Geometry: final body of the model. Coordinates: model frame, mm. A direction names the side the tool comes from. Coordinates: 2 decimals unless noted, no trailing zeros. Write each loop counter-clockwise with the first axis right and the second up, starting at its lowest first coordinate (ties: lowest second). Pieces come first, ordered by that corner, then holes.
from build123d import *

# Parameters (mm, degrees)
ESQUISSE1_R                  = 4
BOSS_EXTRU_1_DEPTH           = 4
ESQUISSE2_R                  = 11
BOSS_EXTRU_2_DEPTH           = 5
ESQUISSE3_R                  = 2.1
ENL_V_MAT_EXTRU_1_DEPTH      = 18.972200756
TROU_TARAUD_M41_D            = 3.3
ESQUISSE6_R                  = 1.25
ENL_V_MAT_EXTRU_2_DEPTH      = 18.972200756
R_P_TITION_CIRCULAIRE1_COUNT = 2
R_P_TITION_CIRCULAIRE1_ANGLE = 90
CHANFREIN1_SIZE              = 0.5


with BuildPart() as part:
    # Esquisse1 → Boss.-Extru.1 (new body)
    with BuildSketch(Plane.XY):
        Circle(ESQUISSE1_R)
    extrude(amount=BOSS_EXTRU_1_DEPTH)

    # Esquisse2 → Boss.-Extru.2 (add)
    with BuildSketch(Plane.XY.offset(4)):
        Circle(ESQUISSE2_R)
    extrude(amount=BOSS_EXTRU_2_DEPTH)

    # Esquisse3 → Enlèv. mat.-Extru.1 (cut, through all)
    with BuildSketch(Plane.XY.offset(9)):
        with Locations((-5.656854249, 5.656854249)):
            Circle(ESQUISSE3_R)
        with Locations((5.656854249, -5.656854249)):
            Circle(ESQUISSE3_R)
        Circle(ESQUISSE3_R)
    extrude(amount=-ENL_V_MAT_EXTRU_1_DEPTH, mode=Mode.SUBTRACT)

    # Trou taraudé M41 (through all)
    with Locations(Plane.XY.offset(9)):
        with Locations((5.656854249, 5.656854249), (-5.656854249, -5.656854249)):
            Hole(TROU_TARAUD_M41_D / 2)

    # Esquisse6 → Enlèv. mat.-Extru.2 (cut, through all)
    with BuildSketch(Plane(origin=(0, 0, 0), x_dir=(1, 0, 0), z_dir=(0, 1, 0))):
        with Locations(Location((0, -6.5, 0), (0, 0, 270))):
            Circle(ESQUISSE6_R)
    enl_v_mat_extru_2 = extrude(amount=-ENL_V_MAT_EXTRU_2_DEPTH, mode=Mode.SUBTRACT)

    # Répétition circulaire1: Enlèv. mat.-Extru.2 ×2 about axis
    r_p_tition_circulaire1_axis = Axis((0, 0, 9), (0, 0, 1))
    for i in range(1, R_P_TITION_CIRCULAIRE1_COUNT):
        add(enl_v_mat_extru_2.rotate(r_p_tition_circulaire1_axis, i * R_P_TITION_CIRCULAIRE1_ANGLE / (R_P_TITION_CIRCULAIRE1_COUNT - 1)), mode=Mode.SUBTRACT)

    # Chanfrein1
    chanfrein1_edges = [part.edges().sort_by_distance(p)[0] for p in [
        (-4, 0, 0),
        (-11, 0, 4),
        (-11, 0, 9),
    ]]
    chamfer(chanfrein1_edges, length=CHANFREIN1_SIZE)


solid = part.part
Item 1: Material intervals for probe 1 along Y at (x, z) = (0, 3.25); probe 2 along X at (y, z) = (-5.75, 5); probe 3 along Y at (x, z) = (-6, 5.5), sorted ascending.
Derived:
probe 1: y = -4 to -2.1, 2.1 to 4
probe 2: x = -9.38 to -7.3, -4.01 to 3.56, 7.75 to 9.38
probe 3: y = -9.22 to -7.27, -4.04 to 3.59, 7.73 to 9.22
Item 2: Pull-direction query (X, two-part tool) for faces 1 (the cylindrical face through (-2.38, -10.74, 6.47)), 2 (the cylindrical face through (5.202, -7.707, 6.535)), 3 (the flat face through (2, -2, 0)); classes: released by +X, released by -X, zero draft, split by the parting line, or undercut.
Derived:
face 1: split by the parting line
face 2: undercut
face 3: zero draft
Item 3: Section D-D, the plane z = 2.5. Output: boundary loops of the cut face in (x, y), plus the area to 3 significant figures.
Derived:
outline: circle Ø8 at (0, 0); hole circle Ø4.2 at (0, 0)
area: 36.4 mm2
Item 4: Pin query (flat end, axial travel): pin 1 (2 mm diameter, centred on x = 0, z = 6.5, fed in from -Y); pin 2 (5 mm diameter, centred on y = -6, z = 3.5, fed in from -X); pin 3 (1 mm diameter, centred on x = -6.5, y = 0.5, fed in from -Z). Return the tip coordinate at first contact, or that it passes through.
Derived:
pin 1: stops at y = 1.85
pin 2: stops at x = -10.36
pin 3: stops at z = 4
Item 5: Set-up query: faces 4 (the flat face through (-0.1, 2.5, 9)), 5 (the cylindrical face through (6.28, 0.05, 5.25)), 6 (the cylindrical face through (-0.867, -3.905, 2.226)), 7 (the cylindrical face through (-7.18, -6.29, 6.46)), 8 (the cylindrical face through (0.05, -6.28, 5.25)). Return all of +Z, -Z, +X, -X, +Y, -Y with unobstructed straight access to the full face (end or side cutting, diameter ignored); none if empty.
Derived:
face 4: +Z, +X, -X, +Y, -Y
face 5: +X
face 6: -Z
face 7: +Z, -Z
face 8: -Y
Item 6: Section B-B, the plane z = 6.5. Output: boundary loops of the cut face in (x, y), plus the area to 3 significant figures.
Derived:
outline: (-1.25, -10.93) - (-1.25, -1.69) arc R2.1 cw (long way) to (1.69, 1.25) - (10.93, 1.25) arc R11 ccw (long way) to start; (1.25, -10.93) arc R11 ccw to (10.93, -1.25) - (1.69, -1.25) arc R2.1 cw to (1.25, -1.69) - close; hole circle Ø4.2 at (-5.66, 5.66); hole circle Ø3.3 at (-5.66, -5.66); hole circle Ø4.2 at (5.66, -5.66); hole circle Ø3.3 at (5.66, 5.66)
area: 276 mm2
Item 7: Section C-C, the plane y = 0. Output: boundary loops of the cut face in (x, z), plus the area to 3 significant figures.
Derived:
outline: (-11, 4.5) - (-10.5, 4) - (-4, 4) - (-4, 0.5) - (-3.5, 0) - (-2.1, 0) - (-2.1, 9) - (-10.5, 9) - (-11, 8.5) - close; (2.1, 0) - (3.5, 0) - (4, 0.5) - (4, 4) - (10.5, 4) - (11, 4.5) - (11, 5.25) - (2.1, 5.25) - close; (2.1, 7.75) - (11, 7.75) - (11, 8.5) - (10.5, 9) - (2.1, 9) - close
area: 81.2 mm2
Item 8: Section A-A, the plane x = 0. Output: boundary loops of the cut face in (y, z), plus the area to 3 significant figures.
Derived:
outline: (-11, 4.5) - (-10.5, 4) - (-4, 4) - (-4, 0.5) - (-3.5, 0) - (-2.1, 0) - (-2.1, 5.25) - (-11, 5.25) - close; (-11, 7.75) - (-2.1, 7.75) - (-2.1, 9) - (-10.5, 9) - (-11, 8.5) - close; (2.1, 0) - (3.5, 0) - (4, 0.5) - (4, 4) - (10.5, 4) - (11, 4.5) - (11, 8.5) - (10.5, 9) - (2.1, 9) - close
area: 81.2 mm2
